The model under review builds one solid part; all positions refer to its coordinate system, in mm. A direction names the side the tool comes from. Round coordinates to 2 decimals unless told otherwise and drop trailing zeros. Order: outer loops, then holes, each group sorted by start corner. A loop starts at its lowest first (then second) coordinate and runs counter-clockwise, first axis right, second up.
1) Machinability: for faces 4 (the face through (3, 0, 0)), 5 (the face through (2.94, 9.12, 0.99)), which of the approach directions +Z, -Z, +X, -X, +Y, -Y give a long, thin tool a straight path to every point of the face, cutting with its end or side? Answer none if there is none.
2) To check wall thickness, follow L1, parallel to Y at x = 0, z = 1.45; L2, parallel to X at y = 6, z = 0.75; L3, parallel to X at y = 7.25, z = 1.75. State the ranges of each line that lie inside material, in increasing order.
3) Consider section A-A (y = 0). Give the boundary of the cut face in (x, z), then the cut area to 3 significant figures.
4) Mouldability with a two-part tool opening along X and no side actions: class faces 1 (the face through (2.95, 2.95, 2)), 2 (the face through (3.07, 3.1, 1.01)), 3 (the face through (1.627, -12.394, 1.014)) as pulls with the +X half, pulls with the -X half, needs draft (parallel to the pull), parting line crosses it, or undercut.
5) Consider section C-C (y = 10). Give the boundary of the cut face in (x, z), then the cut area to 3 significant figures.
6) Clearance check with flat-ended pins moving along their axes: P1, Ø1.6, axis at y = 6, z = 1, coming from the +X side; P2, Ø1.6, axis at x = 7, z = 0.5, coming from the -Y side; P3, Ø1, axis at x = -7, z = 1, coming from the +Y side; P4, Ø1.8, axis at x = 0, y = 0, coming from the +Z side. State where each tip first meets the part, or that it passes through.
Autodesk Inventor part; units mm, degrees
ref_plane "YZ Plane" through (0, 0, 0) normal (1, 0, 0) x (0, 1, 0)
ref_plane "XZ Plane" through (0, 0, 0) normal (0, 1, 0) x (-1, 0, 0)
ref_plane "XY Plane" through (0, 0, 0) normal (0, 0, 1) x (1, 0, 0)
sketch "Sketch1" plane through (0, 0, 0) normal (0, 0, 1) x (1, 0, 0)
  circle A0 centre (-10, 0) radius 1
  circle A1 centre (0, 10) radius 1
  circle A2 centre (0, -10) radius 1
  circle A3 centre (10, 0) radius 1
  circle A4 centre (0, 0) radius 1.5
  arc A5 (10.8355, 3.8525) -> (3.8525, 10.8355) centre (0, 0) ccw
  arc A6 (9.4222, 1.85) -> (10.8355, 3.8525) centre (9.4222, 3.35) ccw
  line L0 (9.4222, 1.85) -> (3.35, 1.85)
  arc A7 (1.85, 3.35) -> (3.35, 1.85) centre (3.35, 3.35) ccw
  line L1 (1.85, 3.35) -> (1.85, 9.4222)
  arc A8 (3.8525, 10.8355) -> (1.85, 9.4222) centre (3.35, 9.4222) ccw
  line L2 (-1.85, 9.4222) -> (-1.85, 3.35)
  arc A9 (-3.35, 1.85) -> (-1.85, 3.35) centre (-3.35, 3.35) ccw
  line L3 (-3.35, 1.85) -> (-9.4222, 1.85)
  arc A10 (-10.8355, 3.8525) -> (-9.4222, 1.85) centre (-9.4222, 3.35) ccw
  arc A11 (-3.8525, 10.8355) -> (-10.8355, 3.8525) centre (0, 0) ccw
  arc A12 (-1.85, 9.4222) -> (-3.8525, 10.8355) centre (-3.35, 9.4222) ccw
  line L4 (3.35, -1.85) -> (9.4222, -1.85)
  arc A13 (10.8355, -3.8525) -> (9.4222, -1.85) centre (9.4222, -3.35) ccw
  arc A14 (3.8525, -10.8355) -> (10.8355, -3.8525) centre (0, 0) ccw
  arc A15 (1.85, -9.4222) -> (3.8525, -10.8355) centre (3.35, -9.4222) ccw
  line L5 (1.85, -9.4222) -> (1.85, -3.35)
  arc A16 (3.35, -1.85) -> (1.85, -3.35) centre (3.35, -3.35) ccw
  line L6 (-1.85, -3.35) -> (-1.85, -9.4222)
  arc A17 (-3.8525, -10.8355) -> (-1.85, -9.4222) centre (-3.35, -9.4222) ccw
  arc A18 (-10.8355, -3.8525) -> (-3.8525, -10.8355) centre (0, 0) ccw
  arc A19 (-9.4222, -1.85) -> (-10.8355, -3.8525) centre (-9.4222, -3.35) ccw
  line L7 (-9.4222, -1.85) -> (-3.35, -1.85)
  arc A20 (-1.85, -3.35) -> (-3.35, -1.85) centre (-3.35, -3.35) ccw
  circle A21 centre (0, 0) radius 12.55
  line L8 (0, -10) -> (0, 10) construction
  line L9 (2.5, -10) -> (2.5, 10)
  line L10 (-2.5, 10) -> (-2.5, -10)
  arc A22 (-2.5, -10) -> (2.5, -10) centre (0, -10) ccw
  arc A23 (2.5, 10) -> (-2.5, 10) centre (0, 10) ccw
  line L11 (10, 0) -> (-10, 0) construction
  line L12 (10, 2.5) -> (-10, 2.5)
  line L13 (-10, -2.5) -> (10, -2.5)
  arc A24 (10, -2.5) -> (10, 2.5) centre (10, 0) ccw
  arc A25 (-10, 2.5) -> (-10, -2.5) centre (-10, 0) ccw
  point P0 (0, 0)
  point P1 (0, 0)
  point P2 (0, 0)
  point P3 (-2.5, -2.5)
  point P4 (2.5, -2.5)
  point P5 (2.5, 2.5)
  point P6 (-2.5, 2.5)
  dimension "d15" = 1
  dimension "d0" = 5
  dimension "d1" = 5
extrude "Extrusion1" add sketch "Sketch1" along normal blind 2 contours A0 | A1 | A2 | A3 | A4 | A24 A13 L4 A16 L9 A7 L0 A6 | A6 L0 A7 L9 L12 A24 | A23 L9 L12 A7 L1 A8 | A8 L1 A7 L12 A9 L2 A12 A23 | A24 L13 L9 A16 L4 A13 | A12 L2 A9 L12 L10 A23 | L9 A7 L12 | L9 A16 L13 A20 L10 A9 L12 A7 | L13 A16 L9 | L9 A22 A15 L5 A16 L13 | L12 A9 L10 | L10 A9 L3 A10 A25 L12 | A22 A17 L6 A20 L13 A16 L5 A15 | A10 L3 A9 L10 A20 L7 A19 A25 | A22 L10 L13 A20 L6 A17 | L13 L10 A20 | A19 L7 A20 L10 L13 A25
sketch "Sketch2" plane through (0, 0, 2) normal (0, 0, 1) x (1, 0, 0)
  line L0 (-2.5, -2.5) -> (-2.5, -10)
  arc A0 (-2.5, -10) -> (2.5, -10) centre (0, -10) ccw
  line L1 (2.5, -10) -> (2.5, -2.5)
  line L2 (2.5, -2.5) -> (10, -2.5)
  arc A1 (10, -2.5) -> (10, 2.5) centre (10, 0) ccw
  line L3 (10, 2.5) -> (2.5, 2.5)
  line L4 (2.5, 2.5) -> (2.5, 10)
  arc A2 (2.5, 10) -> (-2.5, 10) centre (0, 10) ccw
  line L5 (-2.5, 10) -> (-2.5, 2.5)
  line L6 (-2.5, 2.5) -> (-10, 2.5)
  arc A3 (-10, 2.5) -> (-10, -2.5) centre (-10, 0) ccw
  line L7 (-10, -2.5) -> (-2.5, -2.5)
  point P0 (0, 0)
hole "Hole1" at (0, -10, 2) at (10, 0, 2) at (0, 10, 2) at (-10, 0, 2) direction (0, 0, -1) diameter 2 depth 5
sketch "Sketch3" plane through (0, 0, 2) normal (0, 0, 1) x (1, 0, 0)
  circle A0 centre (0, 0) radius 3
  dimension "d11" = 6
extrude "Extrusion2" add sketch "Sketch3" along normal blind 6
fillet "Fillet1" radius 2 4 edges at (2.5, -2.5, 1) (-2.5, -2.5, 1) (-2.5, 2.5, 1) (2.5, 2.5, 1)
fillet "Fillet2" radius 1 1 edges at (-3, 0, 2)
sketch "Sketch4" plane through (0, 0, 8) normal (0, 0, 1) x (1, 0, 0)
  circle A0 centre (0, 0) radius 1
  dimension "d16" = 2
extrude "Extrusion3" cut sketch "Sketch4" against normal blind 12
sketch "Sketch5" plane through (0, 0, 2) normal (0, 0, 1) x (1, 0, 0)
  arc A0 (2.5, 10) -> (-2.5, 10) centre (0, 10) ccw
  line L0 (-2.5, 10) -> (-2.5, 4.5)
  arc A1 (-4.5, 2.5) -> (-2.5, 4.5) centre (-4.5, 4.5) ccw
  line L1 (-4.5, 2.5) -> (-10, 2.5)
  arc A2 (-10, 2.5) -> (-10, -2.5) centre (-10, 0) ccw
  line L2 (-10, -2.5) -> (-4.5, -2.5)
  arc A3 (-2.5, -4.5) -> (-4.5, -2.5) centre (-4.5, -4.5) ccw
  line L3 (-2.5, -4.5) -> (-2.5, -10)
  arc A4 (-2.5, -10) -> (2.5, -10) centre (0, -10) ccw
  line L4 (2.5, -10) -> (2.5, -4.5)
  arc A5 (4.5, -2.5) -> (2.5, -4.5) centre (4.5, -4.5) ccw
  line L5 (4.5, -2.5) -> (10, -2.5)
  arc A6 (10, -2.5) -> (10, 2.5) centre (10, 0) ccw
  line L6 (10, 2.5) -> (4.5, 2.5)
  arc A7 (2.5, 4.5) -> (4.5, 2.5) centre (4.5, 4.5) ccw
  line L7 (2.5, 4.5) -> (2.5, 10)
  circle A8 centre (-10, 0) radius 1
  circle A9 centre (10, 0) radius 1
  circle A10 centre (0, -10) radius 1
  circle A11 centre (0, 10) radius 1
  circle A12 centre (0, 0) radius 4
  circle A13 centre (0, 0) radius 1
  circle A14 centre (0, 0) radius 12.5
  circle A15 centre (0, 0) radius 10
  point P0 (-2.5, -9.6825)
  point P1 (-9.6825, -2.5)
  point P2 (-12.5, 0)
  point P3 (0, -12.5)
  dimension "d19" = 25
  dimension "d20" = 20
extrude "Extrusion4" add sketch "Sketch5" against normal blind 2 contours A2 L2 A15 L3 A4 A14
pattern_circular "Circular Pattern1" count 4 over 360 about axis through (0, 0, 2) along (0, 0, 1) of "Extrusion4"
fillet "Fillet3" radius 1 8 edges at (-2.5, -9.6825, 1) (-9.6825, -2.5, 1) (-9.6825, 2.5, 1) (-2.5, 9.6825, 1) (2.5, 9.6825, 1) (9.6825, 2.5, 1) (9.6825, -2.5, 1) (2.5, -9.6825, 1)
properties part number "tendon_wh_1"
Answer below:
1. face 4: -Z, +X, -X, +Y, -Y
1. face 5: +Z, -Z
2. L1: y = -12.5 to -11, -9 to -1, 1 to 9, 11 to 12.5
2. L2: x = -10.97 to -8, -2.5 to 2.5, 8 to 10.97
2. L3: x = -10.18 to -6.89, -2.5 to 2.5, 6.89 to 10.18
3. outline: (-12.5, 0) - (-11, 0) - (-11, 2) - (-12.5, 2) - close; (-9, 0) - (-1, 0) - (-1, 8) - (-3, 8) - (-3, 3) arc R1 cw to (-4, 2) - (-9, 2) - close; (1, 0) - (9, 0) - (9, 2) - (4, 2) arc R1 cw to (3, 3) - (3, 8) - (1, 8) - close; (11, 0) - (12.5, 0) - (12.5, 2) - (11, 2) - close
3. area: 62.4 mm2
4. face 1: needs draft
4. face 2: undercut
4. face 3: parting line crosses it
5. outline: (-7.5, 0) - (-1, 0) - (-1, 2) - (-7.5, 2) - close; (1, 0) - (7.5, 0) - (7.5, 2) - (1, 2) - close
5. area: 26.0 mm2
6. P1: stops at x = 11.37
6. P2: stops at y = -10.85
6. P3: stops at y = 10.68
6. P4: passes through
